Verification items for the finished model (mm, model axes). A direction names the side the tool comes from. Give positions to 0.01 mm unless a question says otherwise; leave off trailing zeros. Loops run counter-clockwise (first coordinate to the right, second up) from the corner with the lowest first, then second, coordinate; pieces in that order, holes last. Notation, with made-up numbers: (-35.5, 79.5) - (-24.5, 79.5) arc R28 cw to (-24.5, 97.5) - close; hole circle Ø10 at (46, 9.25). An arc over 180 degrees is marked (long way). One line per item, written item: value. Start each with the question number.
1. Sectioned sample at D-D (x = 18). Record the cut outline in (y, z), plus the area to 3 significant figures.
2. Scan lines: L1, parallel to X at y = 6.5, z = -5.25; L2, parallel to Y at x = -26, z = -5.4; L3, parallel to Y at x = -18.5, z = -0.5. Record each from-to range of solid material in increasing order. Write a range as [from, to].
3. Sectioned sample at C-C (y = 7.25). Record the cut outline in (x, z), plus the area to 3 significant figures.
4. Access from +Z, -Z, +X, -X, +Y, -Y to the whole of each face (thin tool, end or side, straight path). Record for faces 5 (the flat face through (2.896, 8, -3)), 6 (the cylindrical face through (21.49, -4.36, -2.96)).
5. Sectioned sample at B-B (y = -1). Record the cut outline in (x, z), plus the area to 3 significant figures.
6. Sectioned sample at A-A (z = -1.5). Record the cut outline in (x, y).
7. Mould release check, pull along X, two halves, no side actions. Record for faces 1 (the cylindrical face through (-28.164, -4.294, -2.958)), 2 (the cylindrical face through (21.555, 11.301, -2.958)), 3 (the cylindrical face through (-23.68, -0.99, -2.96)), 4 (the flat face through (-4, 0, -6)): pulls with the +X half, pulls with the -X half, needs draft (parallel to the pull), parting line crosses it, or undercut.
Autodesk Inventor part; units mm, degrees
ref_plane "YZ Plane" through (0, 0, 0) normal (1, 0, 0) x (0, 1, 0)
ref_plane "XZ Plane" through (0, 0, 0) normal (0, 1, 0) x (-1, 0, 0)
ref_plane "XY Plane" through (0, 0, 0) normal (0, 0, 1) x (1, 0, 0)
sketch "Sketch1" plane through (0, 0, 0) normal (0, 0, 1) x (1, 0, 0)
  circle A0 centre (18.6957, -1.4966) radius 1.7
  circle A1 centre (18.6957, 6.5034) radius 1.7
  circle A2 centre (11.6957, 6.5034) radius 1.7
  arc A3 (22.6957, 8.5034) -> (18.6957, 12.5034) centre (18.6957, 8.5034) ccw
  line L0 (4.8957, 12.5034) -> (18.6957, 12.5034)
  arc A4 (4.8957, 12.5034) -> (2.8957, 10.5034) centre (4.8957, 10.5034) ccw
  line L1 (2.8957, 6.5034) -> (2.8957, 10.5034)
  arc A5 (-9.5043, 6.5034) -> (2.8957, 6.5034) centre (-3.3043, 6.5034) ccw
  line L2 (-9.5043, 10.5034) -> (-9.5043, 6.5034)
  arc A6 (-9.5043, 10.5034) -> (-11.5043, 12.5034) centre (-11.5043, 10.5034) ccw
  line L3 (22.6957, 8.5034) -> (22.6957, -1.4966)
  arc A7 (18.6957, -5.4966) -> (22.6957, -1.4966) centre (18.6957, -1.4966) ccw
  line L4 (-3.3043, 6.5034) -> (-3.3043, -12.8188) construction
  circle A8 centre (-25.3043, -1.4966) radius 1.7
  circle A9 centre (-25.3043, 6.5034) radius 1.7
  circle A10 centre (-18.3043, 6.5034) radius 1.7
  arc A11 (-25.3043, 12.5034) -> (-29.3043, 8.5034) centre (-25.3043, 8.5034) ccw
  line L5 (-11.5043, 12.5034) -> (-25.3043, 12.5034)
  line L6 (-9.5043, 6.5034) -> (-9.5043, 10.5034)
  arc A12 (-9.5043, 6.5034) -> (2.8957, 6.5034) centre (-3.3043, 6.5034) ccw
  line L7 (-29.3043, 8.5034) -> (-29.3043, -1.4966)
  arc A13 (-29.3043, -1.4966) -> (-25.3043, -5.4966) centre (-25.3043, -1.4966) ccw
  line L8 (-25.3043, -5.4966) -> (18.6957, -5.4966)
  point P0 (0, 0)
  dimension "d18" = 4
  dimension "d24" = 6
  dimension "d26" = 2
  dimension "d27" = 2
  dimension "d28" = 2
extrude "Extrusion1" add sketch "Sketch1" against normal blind 6
sketch "Sketch2" plane through (0, 0, -6) normal (0, 0, -1) x (-1, 0, 0)
  circle A0 centre (26.3043, -2.4966) radius 1.6
  circle A1 centre (26.3043, 15.5034) radius 1.6
  circle A2 centre (26.3043, 6.5034) radius 2.5
  arc A3 (30.3043, 15.5034) -> (23.3147, 18.1609) centre (26.3043, 15.5034) ccw
  circle A4 centre (18.3043, 6.5034) radius 1.7
  circle A5 centre (18.3043, -5.4966) radius 1.7
  circle A6 centre (26.3043, -2.4966) radius 1.6
  circle A7 centre (26.3043, 15.5034) radius 1.6
  line L0 (14.3043, 6.5034) -> (14.3043, -5.4966)
  arc A8 (14.3043, -5.4966) -> (19.7088, -9.2419) centre (18.3043, -5.4966) ccw
  line L1 (19.7088, -9.2419) -> (27.7088, -6.2419)
  arc A9 (27.7088, -6.2419) -> (30.3043, -2.4966) centre (26.3043, -2.4966) ccw
  line L2 (30.3043, -2.4966) -> (30.3043, 2.0313)
  arc A10 (30.3043, 2.0313) -> (30.3043, 10.9756) centre (26.3043, 6.5034) ccw
  line L3 (30.3043, 10.9756) -> (30.3043, 15.5034)
  arc A11 (30.3043, 15.5034) -> (23.3147, 18.1609) centre (26.3043, 15.5034) ccw
  line L4 (23.3147, 18.1609) -> (15.3147, 9.1609)
  arc A12 (15.3147, 9.1609) -> (14.3043, 6.5034) centre (18.3043, 6.5034) ccw
  line L5 (18.3043, 12.5242) -> (23.3147, 18.1609) construction
  arc A13 (27.7088, -6.2419) -> (18.3043, -5.4966) centre (19.7185, -47.358) ccw
  line L6 (23.3147, 18.1609) -> (16.508, 12.5034)
  line L7 (-4.8957, 12.5034) -> (-18.6957, 12.5034)
  line L8 (21.8043, 16.9055) -> (21.8043, -5.5246)
  line L9 (25.163, -7.1966) -> (21.8043, -5.5246)
  circle A14 centre (18.3043, 6.5034) radius 1.7
  point P0 (0, 0)
  dimension "d22" = 3.5
sketch "Sketch4" plane through (0, 0, -6) normal (0, 0, -1) x (-1, 0, 0)
  circle A0 centre (-11.6957, 6.5034) radius 1.7
  circle A1 centre (18.3043, 6.5034) radius 1.7
  line L0 (-8.4337, 6.5034) -> (-10.0647, 3.6784)
  line L1 (-10.0647, 3.6784) -> (-13.3267, 3.6784)
  line L2 (-13.3267, 3.6784) -> (-14.9577, 6.5034)
  line L3 (-14.9577, 6.5034) -> (-13.3267, 9.3284)
  line L4 (-13.3267, 9.3284) -> (-10.0647, 9.3284)
  line L5 (-10.0647, 9.3284) -> (-8.4337, 6.5034)
  line L6 (15.0423, 6.5034) -> (16.6733, 9.3284)
  line L7 (16.6733, 9.3284) -> (19.9353, 9.3284)
  line L8 (19.9353, 9.3284) -> (21.5663, 6.5034)
  line L9 (21.5663, 6.5034) -> (19.9353, 3.6784)
  line L10 (19.9353, 3.6784) -> (16.6733, 3.6784)
  line L11 (16.6733, 3.6784) -> (15.0423, 6.5034)
  dimension "d21" = 5.65
properties part number "Extruder_Fixer_normal"
Results are:
1. outline: (-5.5, -6) - (-3.05, -6) - (-3.05, 0) - (-5.5, 0) - close; (0.05, -6) - (4.95, -6) - (4.95, 0) - (0.05, 0) - close; (8.05, -6) - (12.5, -6) - (12.5, 0) - (8.05, 0) - close
1. area: 70.8 mm^2
2. L1: x = [-29.3, -27], [-23.6, -20], [-16.6, -9.5], [2.9, 10], [13.4, 17], [20.4, 22.7]
2. L2: y = [-5.44, -3.05], [0.05, 4.95], [8.05, 12.44]
2. L3: y = [-5.5, 4.81], [8.19, 12.5]
3. outline: (-29.3, -6) - (-26.83, -6) - (-26.83, 0) - (-29.3, 0) - close; (-23.78, -6) - (-19.83, -6) - (-19.83, 0) - (-23.78, 0) - close; (-16.78, -6) - (-9.5, -6) - (-9.5, 0) - (-16.78, 0) - close; (2.9, -6) - (10.17, -6) - (10.17, 0) - (2.9, 0) - close; (13.22, -6) - (17.17, -6) - (17.17, 0) - (13.22, 0) - close; (20.22, -6) - (22.7, -6) - (22.7, 0) - (20.22, 0) - close
3. area: 164 mm^2
4. face 5: +Z, -Z, +Y
4. face 6: +Z, -Z, +X, -Y
5. outline: (-29.3, -6) - (-26.93, -6) - (-26.93, 0) - (-29.3, 0) - close; (-23.68, -6) - (17.07, -6) - (17.07, 0) - (-23.68, 0) - close; (20.32, -6) - (22.7, -6) - (22.7, 0) - (20.32, 0) - close
5. area: 273 mm^2
6. outline: (-29.3, -1.5) arc R4 ccw to (-25.3, -5.5) - (18.7, -5.5) arc R4 ccw to (22.7, -1.5) - (22.7, 8.5) arc R4 ccw to (18.7, 12.5) - (4.9, 12.5) arc R2 ccw to (2.9, 10.5) - (2.9, 6.5) arc R6.2 cw to (-9.5, 6.5) - (-9.5, 10.5) arc R2 ccw to (-11.5, 12.5) - (-25.3, 12.5) arc R4 ccw to (-29.3, 8.5) - close; hole circle Ø3.4 at (-25.3, -1.5); hole circle Ø3.4 at (-25.3, 6.5); hole circle Ø3.4 at (-18.3, 6.5); hole circle Ø3.4 at (11.7, 6.5); hole circle Ø3.4 at (18.7, -1.5); hole circle Ø3.4 at (18.7, 6.5)
7. face 1: pulls with the -X half
7. face 2: pulls with the +X half
7. face 3: undercut
7. face 4: needs draft
